The model under review builds one solid part; all positions refer to its coordinate system, in mm. Coordinates: 2 decimals unless noted, no trailing zeros. Order: outer loops, then holes, each group sorted by start corner. A loop starts at its lowest first (then second) coordinate and runs counter-clockwise, first axis right, second up.
Autodesk Inventor part; units mm, degrees
ref_plane "YZ Plane" through (0, 0, 0) normal (1, 0, 0) x (0, 1, 0)
ref_plane "XZ Plane" through (0, 0, 0) normal (0, 1, 0) x (-1, 0, 0)
ref_plane "XY Plane" through (0, 0, 0) normal (0, 0, 1) x (1, 0, 0)
sketch "Sketch1" plane through (0, 0, 0) normal (0, 0, 1) x (1, 0, 0)
  circle A0 centre (0, 0) radius 6
  circle A1 centre (0, 0) radius 4.4
  dimension "d0" = 12
  dimension "d1" = 8.8
extrude "Extrusion1" add sketch "Sketch1" against normal blind 1.5 contours A0 | A1
extrude "Extrusion2" add sketch "Sketch1" along normal blind 3 draft -10 contours A1
hole "Hole1" at (0, 0, 3) direction (0, 0, -1) diameter 3.5 end through all
properties part number "segment1_coupler1" material "ABS Plastic"
(1) We need section C-C, the plane z = 2.7. Write out the cut boundary in (x, y), and give its area (3 significant figures).
A:
outline: circle Ø7.85 at (0, 0); hole circle Ø3.5 at (0, 0)
area: 38.8 mm2
(2) We need section D-D, the plane z = 0.2. Write out the cut boundary in (x, y), and give its area (3 significant figures).
A:
outline: circle Ø8.73 at (0, 0); hole circle Ø3.5 at (0, 0)
area: 50.2 mm2
(3) Draft analysis for pull direction X (two halves, no side actions). For faces 1 (the face through (3, 4, 0)), 2 (the face through (3.836, -1.208, 2.146)), 3 (the face through (0.67, -1.617, 0.719)), state which applies: released by +X, released by -X, zero draft, split by the parting line, or undercut.
A:
face 1: zero draft
face 2: split by the parting line
face 3: undercut
(4) For pin 1 Ø2 at (x, y) = (0, 0) entering from +Z; pin 2 Ø1.5 at (x, z) = (0, 2.5) entering from +Y; pin 3 Ø5 at (x, y) = (-1.5, -4.5) entering from +Z, all flat-tipped, find the tip position at first contact; note any pin that passes through.
A:
pin 1: passes through
pin 2: stops at y = 4.09
pin 3: stops at z = 3
(5) Wall thickness on probe 1 along Z at (x, y) = (-1.75, -5.25); probe 2 along Y at (x, z) = (0, -0.45); probe 3 along X at (y, z) = (0, 1.3): over which ranges is each line inside the solid? List them lowest first.
A:
probe 1: z = -1.5 to 0
probe 2: y = -6 to -1.75, 1.75 to 6
probe 3: x = -4.17 to -1.75, 1.75 to 4.17
(6) We need section A-A, the plane y = 0. Write out the cut boundary in (x, z).
A:
outline: (-6, -1.5) - (-1.75, -1.5) - (-1.75, 3) - (-3.87, 3) - (-4.4, 0) - (-6, 0) - close; (1.75, -1.5) - (6, -1.5) - (6, 0) - (4.4, 0) - (3.87, 3) - (1.75, 3) - close
